Here's how the part is built. I have some questions about the finished solid (model axes, mm). Face numbers are marked on the shaded views. Coordinates: 2 decimals unless noted, no trailing zeros. Write each loop counter-clockwise with the first axis right and the second up, starting at its lowest first coordinate (ties: lowest second). Pieces come first, ordered by that corner, then holes.
Item 1: If I drill on line 1 (Z direction, x = 45, y = 0); line 2 (X direction, y = -0.5, z = -16); line 3 (X direction, y = 14.5, z = -59), over which ranges is the centre line in solid material (lowest first)?
Item 2: If we section it at C-C (x = 17): Please give me the cut outline in (y, z), then the cut area to 3 significant figures.
Item 3: If we section it at B-B (z = 2): Please give me the cut outline in (x, y), then the cut area to 3 significant figures.
Item 4: If we section it at A-A (y = 0): Please give me the cut outline in (x, z).
Item 5: We'd pull the mould along Z, two halves only. Please class the marked faces 1, 2 and 3: +Z half, -Z half, draft (parallel to the pull), parting line (faces both ways), or undercut.
Item 6: I'm going to push flat-ended pins straight in: pin 1 Ø1 at (y, z) = (28.5, -28) entering from +X; pin 2 Ø2 at (x, z) = (-23.5, -30.5) entering from -Y; pin 3 Ø12 at (x, z) = (-14.5, -1) entering from -Y. Where does each tip first touch, or does it pass through?
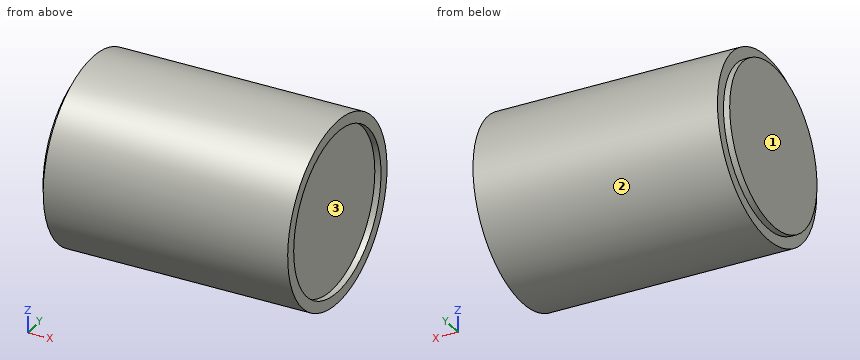
from build123d import *

# Parameters (mm, degrees)
F0_W     = 100.1651920378
F0_H     = 37.5619474798
F3_R     = 33.02
F4_DEPTH = 2.54
F2_R     = 33.02
F5_DEPTH = 2.54


with BuildPart() as f1:
    # F0 (on Front) → F1 (revolve)
    with BuildSketch(Plane.XZ):
        with Locations((-3.2065082341, -8.8560683653)):
            Rectangle(F0_W, F0_H)
    revolve(axis=Axis((-3.2065082341, 0, -27.6370421052), (1, 0, 0)))

    # F3 (on face) → F4 (cut)
    with BuildSketch(Plane.YZ.offset(46.8760877848)):
        with Locations((0, -27.6370421052)):
            Circle(F3_R)
    extrude(amount=-F4_DEPTH, mode=Mode.SUBTRACT)

    # F2 (on face) → F5 (join)
    with BuildSketch(Plane(origin=(-53.2891042531, 0, 0), x_dir=(0, -1, 0), z_dir=(-1, 0, 0))):
        with Locations((0, -27.6370421052)):
            Circle(F2_R)
    extrude(amount=F5_DEPTH)


solid = f1.part
Answer list:
1. line 1: z = -65.2 to -60.66, 5.38 to 9.92
1. line 2: x = -55.83 to 44.34
1. line 3: x = -53.29 to 46.88
2. outline: circle Ø75.12 at (0, -27.64)
2. area: 4,430 mm2
3. outline: (-55.83, -14.56) - (-53.29, -14.56) - (-53.29, -23.08) - (46.88, -23.08) - (46.88, -14.56) - (44.34, -14.56) - (44.34, 14.56) - (46.88, 14.56) - (46.88, 23.08) - (-53.29, 23.08) - (-53.29, 14.56) - (-55.83, 14.56) - close
3. area: 4,620 mm2
4. outline: (-55.83, -60.66) - (-53.29, -60.66) - (-53.29, -65.2) - (46.88, -65.2) - (46.88, -60.66) - (44.34, -60.66) - (44.34, 5.38) - (46.88, 5.38) - (46.88, 9.92) - (-53.29, 9.92) - (-53.29, 5.38) - (-55.83, 5.38) - close
5. face 1: draft
5. face 2: parting line
5. face 3: undercut
6. pin 1: stops at x = 44.34
6. pin 2: stops at y = -37.52
6. pin 3: stops at y = -31.38
